from build123d import *

# Parameters (mm, degrees)
SKETCH1_R               = 3.83
SKETCH1_R_2             = 3.075
BOSS_EXTRUDE1_DEPTH     = 36.5
BOSS_EXTRUDE1_2_DEPTH   = 36.5
BOSS_EXTRUDE1_3_DEPTH   = 36.5
SKETCH2_R               = 3.075
BOSS_EXTRUDE2_DEPTH     = 1.5
SKETCH3_R               = 3.075
BOSS_EXTRUDE3_DEPTH     = 17.2
SKETCH4_R               = 3.075
BOSS_EXTRUDE4_DEPTH     = 2.29
CUT_EXTRUDE1_DEPTH      = 1.4
FILLET1_R               = 0.25
CUT_EXTRUDE_THIN2_DEPTH = 1.6
SKETCH7_W               = 6.15
SKETCH7_H               = 8.738173166
SKETCH7_H_2             = 8.358950775
CUT_EXTRUDE2_DEPTH      = 3


with BuildPart() as part:
    # Sketch1 → Boss-Extrude1 (new body)
    with BuildSketch(Plane(origin=(0, 0, 0), x_dir=(1, 0, 0), z_dir=(0, 1, 0))):
        with Locations(Location((0, 0, 0), (0, 0, 270))):
            Circle(SKETCH1_R)
        with Locations(Location((0, 0, 0), (0, 0, 270))):
            Circle(SKETCH1_R_2, mode=Mode.SUBTRACT)
    extrude(amount=BOSS_EXTRUDE1_DEPTH)



with BuildPart() as body_2:
    # Sketch1 → Boss-Extrude1 2 (new body)
    with BuildSketch(Plane(origin=(0, 0, 0), x_dir=(1, 0, 0), z_dir=(0, 1, 0))):
        with BuildLine():
            Line((-10.06, 3.83), (-13.89, 3.83))
            Line((-13.89, 3.83), (-13.89, -3.83))
            Line((-13.89, -3.83), (-10.06, -3.83))
            ThreePointArc((-10.06, -3.83), (-6.23, 0), (-10.06, 3.83))
        make_face()
        with Locations(Location((-10.06, 0, 0), (0, 0, 270))):
            Circle(SKETCH1_R_2, mode=Mode.SUBTRACT)
    extrude(amount=BOSS_EXTRUDE1_2_DEPTH)


with BuildPart() as body_3:
    # Sketch1 → Boss-Extrude1 3 (new body)
    with BuildSketch(Plane(origin=(0, 0, 0), x_dir=(1, 0, 0), z_dir=(0, 1, 0))):
        with BuildLine():
            Line((10.06, 3.83), (6.23, 3.83))
            Line((6.23, 3.83), (6.23, -3.83))
            Line((6.23, -3.83), (10.06, -3.83))
            ThreePointArc((10.06, -3.83), (13.89, 0), (10.06, 3.83))
        make_face()
        with Locations(Location((10.06, 0, 0), (0, 0, 270))):
            Circle(SKETCH1_R_2, mode=Mode.SUBTRACT)
    extrude(amount=BOSS_EXTRUDE1_3_DEPTH)


with BuildPart() as part_1:
    add(part.part)

    add(body_2.part)  # Boss-Extrude2 merges body 2

    add(body_3.part)  # Boss-Extrude2 merges body 3
    # Sketch2 → Boss-Extrude2 (add)
    with BuildSketch(Plane(origin=(0, 0, 0), x_dir=(1, 0, 0), z_dir=(0, 1, 0))):
        with BuildLine():
            Line((-10.06, 5.85), (10.06, 5.85))
            ThreePointArc((10.06, 5.85), (15.91, 0), (10.06, -5.85))
            Line((10.06, -5.85), (-10.06, -5.85))
            Line((-10.06, -5.85), (-16.09, -5.85))
            Line((-16.09, -5.85), (-16.09, 5.85))
            Line((-16.09, 5.85), (-10.06, 5.85))
        make_face()
        with Locations(Location((-10.06, 0, 0), (0, 0, 270))):
            Circle(SKETCH2_R, mode=Mode.SUBTRACT)
        with Locations(Location((0, 0, 0), (0, 0, 270))):
            Circle(SKETCH2_R, mode=Mode.SUBTRACT)
        with Locations(Location((10.06, 0, 0), (0, 0, 270))):
            Circle(SKETCH2_R, mode=Mode.SUBTRACT)
        with BuildLine():
            Line((5.485, -2.6), (5.485, 2.6))
            Line((5.485, 2.6), (3.764389061, 2.6))
            ThreePointArc((3.764389061, 2.6), (4.575, 0), (3.764389061, -2.6))
            Line((3.764389061, -2.6), (5.485, -2.6))
        make_face(mode=Mode.SUBTRACT)
        with BuildLine():
            Line((-3.764389061, 2.6), (-6.295610939, 2.6))
            ThreePointArc((-6.295610939, 2.6), (-5.485, 0), (-6.295610939, -2.6))
            Line((-6.295610939, -2.6), (-3.764389061, -2.6))
            ThreePointArc((-3.764389061, -2.6), (-4.575, 0), (-3.764389061, 2.6))
        make_face(mode=Mode.SUBTRACT)
    extrude(amount=BOSS_EXTRUDE2_DEPTH)

    # Sketch3 → Boss-Extrude3 (add)
    with BuildSketch(Plane(origin=(0, 1.5, 0), x_dir=(1, 0, 0), z_dir=(0, 1, 0))):
        with BuildLine():
            Line((-1.387862692, -3.83), (-13.89, -3.83))
            Line((-13.89, -3.83), (-13.89, 3.83))
            Line((-13.89, 3.83), (-3.321031177, 3.83))
            Line((-3.321031177, 3.83), (10.06, 3.83))
            ThreePointArc((10.06, 3.83), (13.89, 0), (10.06, -3.83))
            Line((10.06, -3.83), (-1.387862692, -3.83))
        make_face()
        with Locations(Location((-10.06, 0, 0), (0, 0, 270))):
            Circle(SKETCH3_R, mode=Mode.SUBTRACT)
        with Locations(Location((0, 0, 0), (0, 0, 270))):
            Circle(SKETCH3_R, mode=Mode.SUBTRACT)
        with Locations(Location((10.06, 0, 0), (0, 0, 270))):
            Circle(SKETCH3_R, mode=Mode.SUBTRACT)
        with BuildLine():
            Line((-3.764389061, 2.6), (-6.295610939, 2.6))
            ThreePointArc((-6.295610939, 2.6), (-5.485, 0), (-6.295610939, -2.6))
            Line((-6.295610939, -2.6), (-3.764389061, -2.6))
            ThreePointArc((-3.764389061, -2.6), (-4.575, 0), (-3.764389061, 2.6))
        make_face(mode=Mode.SUBTRACT)
        with BuildLine():
            Line((5.485, -2.6), (5.485, 2.6))
            Line((5.485, 2.6), (3.764389061, 2.6))
            ThreePointArc((3.764389061, 2.6), (4.575, 0), (3.764389061, -2.6))
            Line((3.764389061, -2.6), (5.485, -2.6))
        make_face(mode=Mode.SUBTRACT)
    extrude(amount=BOSS_EXTRUDE3_DEPTH)

    # Sketch4 → Boss-Extrude4 (add)
    with BuildSketch(Plane(origin=(0, 18.7, 0), x_dir=(1, 0, 0), z_dir=(0, 1, 0))):
        with BuildLine():
            Line((10.06, 5.85), (-10.06, 5.85))
            Line((-10.06, 5.85), (-16.09, 5.85))
            Line((-16.09, 5.85), (-16.09, -5.85))
            Line((-16.09, -5.85), (-10.06, -5.85))
            Line((-10.06, -5.85), (10.06, -5.85))
            ThreePointArc((10.06, -5.85), (15.91, 0), (10.06, 5.85))
        make_face()
        with Locations(Location((-10.06, 0, 0), (0, 0, 270))):
            Circle(SKETCH4_R, mode=Mode.SUBTRACT)
        with Locations(Location((10.06, 0, 0), (0, 0, 270))):
            Circle(SKETCH4_R, mode=Mode.SUBTRACT)
        with Locations(Location((0, 0, 0), (0, 0, 270))):
            Circle(SKETCH4_R, mode=Mode.SUBTRACT)
        with BuildLine():
            Line((-3.764389061, 2.6), (-6.295610939, 2.6))
            ThreePointArc((-6.295610939, 2.6), (-5.485, 0), (-6.295610939, -2.6))
            Line((-6.295610939, -2.6), (-3.764389061, -2.6))
            ThreePointArc((-3.764389061, -2.6), (-4.575, 0), (-3.764389061, 2.6))
        make_face(mode=Mode.SUBTRACT)
        with BuildLine():
            Line((5.485, -2.6), (5.485, 2.6))
            Line((5.485, 2.6), (3.764389061, 2.6))
            ThreePointArc((3.764389061, 2.6), (4.575, 0), (3.764389061, -2.6))
            Line((3.764389061, -2.6), (5.485, -2.6))
        make_face(mode=Mode.SUBTRACT)
    extrude(amount=BOSS_EXTRUDE4_DEPTH)

    # Sketch5 → Cut-Extrude1 (cut)
    with BuildSketch(Plane.XZ.offset(-18.7)):
        with BuildLine():
            Line((-16.09, 5.85), (10.06, 5.85))
            ThreePointArc((10.06, 5.85), (15.91, 0), (10.06, -5.85))
            Line((10.06, -5.85), (-16.09, -5.85))
            Line((-16.09, -5.85), (-16.09, 5.85))
        make_face()
        with BuildLine():
            Line((-15.09, 4.85), (10.06, 4.85))
            ThreePointArc((10.06, 4.85), (14.91, 0), (10.06, -4.85))
            Line((10.06, -4.85), (-15.09, -4.85))
            Line((-15.09, -4.85), (-15.09, 4.85))
        make_face(mode=Mode.SUBTRACT)
    extrude(amount=-CUT_EXTRUDE1_DEPTH, mode=Mode.SUBTRACT)

    # Fillet1
    fillet1_edges = [part_1.edges().sort_by_distance(p)[0] for p in [
        (-3.764389061, 10.495, -2.6),
        (-6.295610939, 10.495, -2.6),
        (-6.295610939, 10.495, 2.6),
        (-3.764389061, 10.495, 2.6),
        (5.485, 10.495, 2.6),
        (5.485, 10.495, -2.6),
        (3.764389061, 10.495, -2.6),
        (3.764389061, 10.495, 2.6),
    ]]
    fillet(fillet1_edges, radius=FILLET1_R)

    # Sketch6 → Cut-Extrude-Thin2 (cut)
    with BuildSketch(Plane.XZ):
        Polygon((-10.31, 0), (-10.31, -6.991466743), (10.31, -7.436536546), (10.31, 0), (9.81, 0), (9.81, -6.925627901), (-9.81, -6.502142473), (-9.81, 0), align=None)
    extrude(amount=-CUT_EXTRUDE_THIN2_DEPTH, mode=Mode.SUBTRACT)

    # Sketch7 → Cut-Extrude2 (cut)
    with BuildSketch(Plane(origin=(0, 1.5, 0), x_dir=(1, 0, 0), z_dir=(0, 1, 0))):
        with Locations((-10.06, 4.369086583)):
            Rectangle(SKETCH7_W, SKETCH7_H)
        with Locations((10.06, 4.179475388)):
            Rectangle(SKETCH7_W, SKETCH7_H_2)
    extrude(amount=CUT_EXTRUDE2_DEPTH, mode=Mode.SUBTRACT)


solid = part_1.part
Geometry: final body of the model. Coordinates: model frame, mm. A direction names the side the tool comes from. Coordinates: 2 decimals unless noted, no trailing zeros. Write each loop counter-clockwise with the first axis right and the second up, starting at its lowest first coordinate (ties: lowest second). Pieces come first, ordered by that corner, then holes. Notation, with made-up numbers: (-24, 11) - (34, 11) arc R22 ccw to (34, 41) - close; hole circle Ø5 at (83, 4). An arc over 180 degrees is marked (long way). Return JSON: item names as keys, results as strings.
Item 1: Line query: L1, parallel to Z at x = 10.06, y = 23.5 (3 decimals); L2, parallel to X at y = 3, z = 0.25 (3 decimals); L3, parallel to Y at x = -4, z = -5. Output: solid intervals per line, ascending.
Completed:
{"L1": "z = -3.83 to -3.075, 3.075 to 3.83", "L2": "x = -13.89 to -13.125, -6.995 to -5.492, -4.568 to -3.065, 3.065 to 4.568, 5.485 to 6.995, 13.125 to 13.882", "L3": "y = 0 to 1.5, 20.1 to 20.99"}
Item 2: Reachability of faces 1 (the face through (-2, 19, -4.85)), 2 (the face through (14.91, 19.39, 0.11)), 3 (the face through (-1, 20.1, -5)), 4 (the face through (-10.1, 4.5, -3.6)), 5 (the face through (-13.89, 10, 0)) from +Z, -Z, +X, -X, +Y, -Y: full face, straight path, thin tool, end or side. Return the list, or none.
Completed:
{"face 1": "-Z, +X, -X", "face 2": "+X", "face 3": "none", "face 4": "-Z", "face 5": "+Z, -Z, -X"}
Item 3: Pull-direction query (Z, two-part tool) for faces 6 (the face through (-2, 10, 3.83)), 7 (the face through (0, 1.5, -5)), 8 (the face through (5, 10, 2.6)), 9 (the face through (-4.575, 10.348, 0.033)); classes: +Z half, -Z half, draft (parallel to the pull), parting line (faces both ways), or undercut.
Completed:
{"face 6": "+Z half", "face 7": "draft", "face 8": "undercut", "face 9": "undercut"}
Item 4: Section query D-D (y = 7). Output: boundary loops of the cut face in (x, z) (3 decimals).
Completed:
{"outline": "(-13.89, -3.83) - (10.06, -3.83) arc R3.83 ccw to (10.06, 3.83) - (-13.89, 3.83) - close; hole circle Ø6.15 at (-10.06, 0); hole (-6.064, -2.228) arc R0.25 ccw to (-5.846, -2.6) - (-4.214, -2.6) arc R0.25 ccw to (-3.996, -2.228) arc R4.575 cw to (-3.996, 2.228) arc R0.25 ccw to (-4.214, 2.6) - (-5.846, 2.6) arc R0.25 ccw to (-6.064, 2.228) arc R4.575 cw to start; hole circle Ø6.15 at (0, 0); hole (3.996, -2.228) arc R0.25 ccw to (4.214, -2.6) - (5.235, -2.6) arc R0.25 ccw to (5.485, -2.35) - (5.485, 2.35) arc R0.25 ccw to (5.235, 2.6) - (4.214, 2.6) arc R0.25 ccw to (3.996, 2.228) arc R4.575 cw to start; hole circle Ø6.15 at (10.06, 0)"}
Item 5: Pin query (flat end, axial travel): pin 1 Ø2 at (y, z) = (10, 1) entering from +X; pin 2 Ø1.9 at (x, y) = (8.5, 26) entering from +Z; pin 3 Ø2.5 at (y, z) = (28.5, -0.5) entering from -X. Return the tip coordinate at first contact, or that it passes through.
Completed:
{"pin 1": "stops at x = 13.89", "pin 2": "stops at z = 3.83", "pin 3": "stops at x = -13.89"}
Item 6: Section query B-B (x = 0). Output: boundary loops of the cut face in (y, z) (3 decimals), and give its area (3 significant figures).
Completed:
{"outline": "(0, -5.85) - (1.5, -5.85) - (1.5, -3.83) - (18.7, -3.83) - (18.7, -4.85) - (20.1, -4.85) - (20.1, -5.85) - (20.99, -5.85) - (20.99, -3.83) - (36.5, -3.83) - (36.5, -3.075) - (0, -3.075) - close; (0, 3.075) - (36.5, 3.075) - (36.5, 3.83) - (20.99, 3.83) - (20.99, 5.85) - (20.1, 5.85) - (20.1, 4.85) - (18.7, 4.85) - (18.7, 3.83) - (1.5, 3.83) - (1.5, 5.85) - (0, 5.85) - close", "area": "67.6 mm2"}
Item 7: Section query A-A (y = 32). Output: boundary loops of the cut face in (x, z) (3 decimals).
Completed:
{"outline": "(-13.89, -3.83) - (-10.06, -3.83) arc R3.83 ccw to (-10.06, 3.83) - (-13.89, 3.83) - close; circle Ø7.66 at (0, 0); (6.23, -3.83) - (10.06, -3.83) arc R3.83 ccw to (10.06, 3.83) - (6.23, 3.83) - close; hole circle Ø6.15 at (-10.06, 0); hole circle Ø6.15 at (0, 0); hole circle Ø6.15 at (10.06, 0)"}
Item 8: Section query C-C (x = 7.5). Output: boundary loops of the cut face in (y, z).
Completed:
{"outline": "(0, -5.85) - (1.5, -5.85) - (1.5, -1.7) - (0, -1.7) - close; (0, 1.7) - (36.5, 1.7) - (36.5, 3.83) - (20.99, 3.83) - (20.99, 5.85) - (20.1, 5.85) - (20.1, 4.85) - (18.7, 4.85) - (18.7, 3.83) - (1.5, 3.83) - (1.5, 5.85) - (0, 5.85) - close; (4.5, -3.83) - (18.7, -3.83) - (18.7, -4.85) - (20.1, -4.85) - (20.1, -5.85) - (20.99, -5.85) - (20.99, -3.83) - (36.5, -3.83) - (36.5, -1.7) - (4.5, -1.7) - close"}
